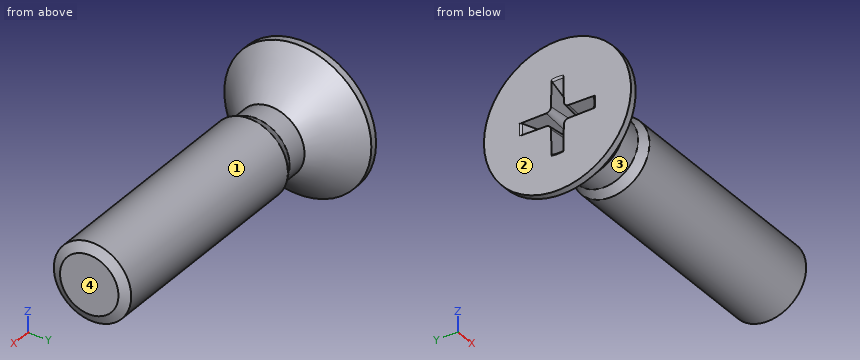
Autodesk Inventor part; units mm, degrees
ref_plane "Work Plane2" through (3.35, 0, 0) normal (0, 0, -1) x (1, 0, 0)
ref_plane "YZ Plane" through (0, 0, 0) normal (1, 0, 0) x (0, 1, 0)
ref_plane "XZ Plane" through (0, 0, 0) normal (0, 1, 0) x (-1, 0, 0)
sketch "Sketch1" plane through (0, 0, 0) normal (0, 0, 1) x (1, 0, 0)
  line L0 (1.2, 0) -> (8, 0)
  line L1 (8, 0) -> (8, 1)
  line L2 (8, 1) -> (2, 1)
  line L3 (2, 1) -> (1.7546, 0.8773)
  line L4 (1.7546, 0.8773) -> (1.2, 0.8773)
  line L5 (0, 1.9) -> (0, 0.95)
  line L6 (0, 0.95) -> (0.9455, 0.4786)
  line L7 (0.9455, 0.4786) -> (1.2, 0)
  line L8 (-1.6, 0) -> (9.6, 0)
  line L9 (0, -0.38) -> (0, 2.28)
  line L10 (0, 1.9) -> (0.1773, 1.9)
  line L11 (0.1773, 1.9) -> (1.2, 0.8773)
  line L12 (2, 1) -> (1.0773, 1) construction
  dimension "d1" = 6
  dimension "d2" = 2
  dimension "d3" = 1.7546
  dimension "d4" = 1.9
  dimension "d5" = 26.5
  dimension "d6" = 62
  dimension "d7" = 1.2
  dimension "d8" = 0.2454
  dimension "d12" = 3.8
  dimension "d13" = 45
  dimension "d15" = 8
  dimension "d24" = 1.2
revolve "Body" add sketch "Sketch1" angle 360 about axis through (1.2, 0, 0) along (1, 0, 0) contours L7 L6 L5 L10 L11 L4 L3 L2 L1 L0
sketch "Sketch2" plane through (0, 0, 0) normal (-1, 0, 0) x (0, 0, 1)
  line L0 (0, 0.95) -> (0, 0) construction
  line L1 (0, 0) -> (0.95, 0) construction
  arc A0 (0.285, 0) -> (0, 0.285) centre (0, 0) ccw construction
  arc A1 (0.3325, 0) -> (0, 0.3325) centre (0, 0) ccw construction
  arc A2 (0.9373, 0.155) -> (0.155, 0.9373) centre (0, 0) ccw
  line L2 (0, 0) -> (0.6718, 0.6718) construction
  line L3 (0.155, 0.9373) -> (0.1646, 0.2889)
  line L4 (0.9373, 0.155) -> (0.2889, 0.1646)
  arc A3 (0.155, 0.9373) -> (0, 0.95) centre (0, 0) ccw
  arc A4 (0.95, 0) -> (0.9373, 0.155) centre (0, 0) ccw
  line L5 (0, -2.66) -> (0, 2.66)
  line L6 (-2.66, 0) -> (2.66, 0)
  arc A5 (0.155, -0.9373) -> (0.9373, -0.155) centre (0, 0) ccw
  line L7 (0.155, -0.9373) -> (0.1646, -0.2889)
  line L8 (0.9373, -0.155) -> (0.2889, -0.1646)
  arc A6 (0, -0.95) -> (0.155, -0.9373) centre (0, 0) ccw
  arc A7 (0.9373, -0.155) -> (0.95, 0) centre (0, 0) ccw
  arc A8 (-0.155, 0.9373) -> (-0.9373, 0.155) centre (0, 0) ccw
  line L9 (-0.155, 0.9373) -> (-0.1646, 0.2889)
  line L10 (-0.9373, 0.155) -> (-0.2889, 0.1646)
  arc A9 (0, 0.95) -> (-0.155, 0.9373) centre (0, 0) ccw
  arc A10 (-0.9373, 0.155) -> (-0.95, 0) centre (0, 0) ccw
  arc A11 (-0.155, -0.9373) -> (0, -0.95) centre (0, 0) ccw
  arc A12 (-0.9373, -0.155) -> (-0.155, -0.9373) centre (0, 0) ccw
  arc A13 (-0.95, 0) -> (-0.9373, -0.155) centre (0, 0) ccw
  line L11 (-0.9373, -0.155) -> (-0.2889, -0.1646)
  line L12 (-0.155, -0.9373) -> (-0.1646, -0.2889)
  arc A14 (0.1646, 0.2889) -> (0.2889, 0.1646) centre (0.2908, 0.2908) ccw
  arc A15 (0.2889, -0.1646) -> (0.1646, -0.2889) centre (0.2908, -0.2908) ccw
  arc A16 (-0.2889, 0.1646) -> (-0.1646, 0.2889) centre (-0.2908, 0.2908) ccw
  arc A17 (-0.1646, -0.2889) -> (-0.2889, -0.1646) centre (-0.2908, -0.2908) ccw
  point P0 (0.6718, -0.6718)
  point P1 (-0.6718, 0.6718)
  point P2 (-0.6718, -0.6718)
  dimension "d17" = 0.57
  dimension "d18" = 0.665
  dimension "d19" = 1.9
  dimension "d20" = 45
  dimension "d21" = 0.155
extrude "Slot" add sketch "Sketch2" against normal up to next draft 5 contours L4 A14 L3 A2 | A5 L7 A15 L8 | L9 A16 L10 A8 | A12 L11 A17 L12
fillet "Fillet1" radius 0.062 4 edges at (0, 0.95, 0) (0, 0, -0.95) (0, -0.95, 0) (0, 0, 0.95)
thread "Thread"
chamfer "Chamfer1" distance 0.2454 distance2 0.1227 1 edges at (8, -1, 0) measured on face at (8, -0.1182, -0.3117)
ref_plane "Work Plane2" through (3.35, 0, 0) normal (0, 0, -1) x (1, 0, 0)
equation "\"d1\" = GEL"
equation "\"d2\" = GD"
equation "\"d3\" = BDM"
equation "\"d4\" = SDM"
equation "\"d7\" = INTI"
equation "\"d8\" = GAL"
equation "\"d12\" = KOD"
equation "\"d13\" = 0.5 * SEWI"
equation "\"d15\" = NLG"
equation "\"d24\" = KOH"
equation "\"d17\" = 0.3 * SDM"
equation "\"d18\" = 0.35 * SDM"
equation "\"d19\" = SDM"
equation "\"d21\" = 0.5 * SBR"
equation "\"d23\" = 0.2 * SBR"
equation "\"d10\" = GEL"
equation "\"d25\" = -0.5 * SPD + 0.5 * GD"
equation "\"d26\" = 0.5 * GAL"
equation "\"NLG\" = 8"
equation "\"GEL\" = 6"
equation "\"GAL\" = 0.61345 * PTC"
equation "\"SPD\" = NND - 1.2269 * PTC"
equation "\"KOD\" = 3.8"
equation "\"KOH\" = 1.2"
equation "\"SBR\" = 0.31"
equation "\"INTI\" = 1.2"
equation "\"SDM\" = 1.9"
equation "\"GD\" = NND"
equation "\"BDM\" = NND - GAL"
equation "\"SEWI\" = 90deg"
equation "\"d9\" = SDM"
equation "\"GUL\" = 0.61345 * PTC"
equation "\"TOA\" = 30deg"
equation "\"EPV\" = 2.2"
equation "\"THREADDIA\" = 2"
equation "\"PTC\" = 0.4"
equation "\"NND\" = 2"
equation "\"GD1\" = THREADDIA - 1.2269 * PTC"
properties part number "ISO 7046-1 - M2 x 8 - 4.8 - H" material "Steel"
Build history of the part. All positions in model axes, mm. Face numbers are marked on the shaded views. Round coordinates to 2 decimals unless told otherwise and drop trailing zeros. Write each loop counter-clockwise with the first axis right and the second up, starting at its lowest first coordinate (ties: lowest second). Pieces come first, ordered by that corner, then holes. Notation, with made-up numbers: M -22,-8.5 L -2,-8.5 A12 ccw -2,-2.5 Z; hole C 13,59.5 d11. An arc over 180 degrees is marked long. Use CSV: the item, a comma, the result in double quotes.
1. Wall check: probe 1 along X at (y, z) = (1.6, 0); probe 2 along X at (y, z) = (-0.3, -1.45); probe 3 along Y at (x, z) = (5.5, 0.4). Give the ranges that are in metal, low to high. Write a range as from..to.
Reply:
probe 1,"x = 0..0.48"
probe 2,"x = 0..0.6"
probe 3,"y = -0.92..0.92"
2. Saw through at A-A (x = 3.75). Give the cut face in (y, z), plus the area to 3 significant figures.
Reply:
outline,"C 0,0 d2"
area,"3.14 mm²"
3. Two-plate mould, pull along X, no slides. Class the marked faces 1, 2, 3 and 4: +X half, -X half, draft (parallel to the pull), parting line (faces both ways), or undercut.
Reply:
face 1,"draft"
face 2,"-X half"
face 3,"undercut"
face 4,"+X half"
4. Flat gauge pin, fed straight in: pin 1 (2 mm diameter, centred on x = 1, z = -1, fed in from +Y). Where does the tip first touch, or does it go through?
Reply:
pin 1,"stops at y = 1.85"
